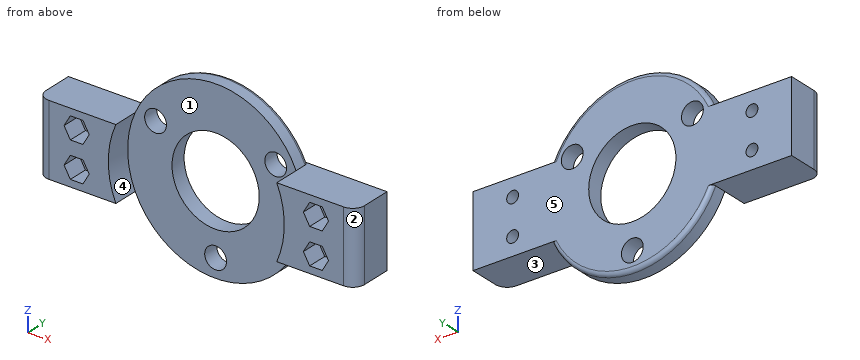
from build123d import *

# Parameters (mm, degrees)
SKETCH1_R                = 17.45
SKETCH1_R_2              = 12.45
BOSS_EXTRUDE1_DEPTH      = 8
SKETCH2_R                = 20
SKETCH2_R_2              = 12.45
BOSS_EXTRUDE2_DEPTH      = 2
SKETCH3_R                = 32.5
SKETCH3_R_2              = 12.45
BOSS_EXTRUDE3_DEPTH      = 4
FILLET1_R                = 1
BOSS_EXTRUDE6_START      = -4
SKETCH10_W               = 10
SKETCH10_H               = 18
BOSS_EXTRUDE6_DEPTH      = 4
SKETCH4_W                = 6
SKETCH4_H                = 18
BOSS_EXTRUDE4_DEPTH      = 75
BOSS_EXTRUDE4_DEPTH_BACK = 4
SKETCH5_R                = 5.05
CUT_EXTRUDE1_DEPTH       = 306
CUT_EXTRUDE1_DEPTH_BACK  = 113
SKETCH6_W                = 6
SKETCH6_H                = 10
BOSS_EXTRUDE5_DEPTH      = 15
BOSS_EXTRUDE5_DEPTH_BACK = 32.85
SKETCH7_R                = 1.629220746
SKETCH7_R_2              = 1.580258945
CUT_EXTRUDE2_DEPTH       = 10
SKETCH9_R                = 5.05
CUT_EXTRUDE3_DEPTH       = 10
CUT_EXTRUDE3_DEPTH_BACK  = 10
SKETCH11_W               = 9.782596874
SKETCH11_H               = 3.234517514
CUT_EXTRUDE4_DEPTH       = 123
CUT_EXTRUDE4_DEPTH_BACK  = 61
FILLET4_R                = 3
FILLET5_R                = 3
SKETCH12_W               = 108.791398151
SKETCH12_H               = 24.041848298
CUT_EXTRUDE5_DEPTH       = 110.678
SKETCH15_R               = 22
CUT_EXTRUDE7_DEPTH       = 4
SKETCH13_R               = 22
SKETCH13_R_2             = 11
SKETCH13_R_3             = 2.75
BOSS_EXTRUDE7_DEPTH      = 4
FILLET6_R                = 3
CUT_EXTRUDE8_DEPTH       = 5
FILLET7_R                = 1
BOSS_EXTRUDE8_START      = -3
BOSS_EXTRUDE8_DEPTH      = 9.4
FILLET8_R                = 3
FILLET8_OF_MIRROR2_R     = 3
CUT_EXTRUDE12_START      = -6
SKETCH21_R               = 6.05
CUT_EXTRUDE12_DEPTH      = 3.8
SKETCH18_W               = 88.746975794
SKETCH18_H               = 20.386854219
CUT_EXTRUDE9_DEPTH       = 10
SKETCH19_W               = 6
SKETCH19_H               = 10.45
BOSS_EXTRUDE9_DEPTH      = 5
FILLET9_R                = 2
CUT_EXTRUDE13_DEPTH      = 2
SKETCH23_R               = 1
CUT_EXTRUDE14_DEPTH      = 11
CUT_EXTRUDE16_DEPTH      = 1.7
SKETCH26_W               = 136.459260558
SKETCH26_H               = 86.542262852
CUT_EXTRUDE17_DEPTH      = 100
CUT_EXTRUDE17_DEPTH_BACK = 100
SKETCH27_R               = 1.5
CUT_EXTRUDE18_DEPTH      = 100
CUT_EXTRUDE19_DEPTH      = 5


with BuildPart() as part:
    # Sketch1 → Boss-Extrude1 (new body)
    with BuildSketch(Plane(origin=(0, 0, 0), x_dir=(1, 0, 0), z_dir=(0, 1, 0))):
        Circle(SKETCH1_R)
        Circle(SKETCH1_R_2, mode=Mode.SUBTRACT)
    extrude(amount=BOSS_EXTRUDE1_DEPTH)

    # Sketch2 → Boss-Extrude2 (add)
    with BuildSketch(Plane(origin=(0, 8, 0), x_dir=(1, 0, 0), z_dir=(0, 1, 0))):
        Circle(SKETCH2_R)
        Circle(SKETCH2_R_2, mode=Mode.SUBTRACT)
    extrude(amount=BOSS_EXTRUDE2_DEPTH)

    # Sketch3 → Boss-Extrude3 (add)
    with BuildSketch(Plane(origin=(0, 10, 0), x_dir=(1, 0, 0), z_dir=(0, 1, 0))):
        Circle(SKETCH3_R)
        Circle(SKETCH3_R_2, mode=Mode.SUBTRACT)
    extrude(amount=BOSS_EXTRUDE3_DEPTH)

    # Fillet1
    fillet1_edges = [part.edges().sort_by_distance(p)[0] for p in [
        (-32.5, 14, 0),
    ]]
    fillet(fillet1_edges, radius=FILLET1_R)

    # Sketch10 → Boss-Extrude6 (add)
    with BuildSketch(Plane(origin=(0, 14, 0), x_dir=(1, 0, 0), z_dir=(0, 1, 0)).offset(BOSS_EXTRUDE6_START)):
        with Locations((35.186917696, 0)):
            Rectangle(SKETCH10_W, SKETCH10_H)
        with Locations((-35.186917696, 0)):
            Rectangle(SKETCH10_W, SKETCH10_H)
    extrude(amount=BOSS_EXTRUDE6_DEPTH)

    # Sketch4 → Boss-Extrude4 (add, two sides)
    with BuildSketch(Plane(origin=(0, 14, 0), x_dir=(1, 0, 0), z_dir=(0, 1, 0))) as boss_extrude4_sk:
        with Locations((-37.186917696, 0)):
            Rectangle(SKETCH4_W, SKETCH4_H)
        with Locations((37.186917696, 0)):
            Rectangle(SKETCH4_W, SKETCH4_H)
    extrude(amount=BOSS_EXTRUDE4_DEPTH)
    extrude(boss_extrude4_sk.sketch, amount=-BOSS_EXTRUDE4_DEPTH_BACK)

    # Sketch5 → Cut-Extrude1 (cut, two sides)
    with BuildSketch(Plane.ZY.offset(-34.186917696)) as cut_extrude1_sk:
        with Locations((0, 79)):
            Circle(SKETCH5_R)
    extrude(amount=CUT_EXTRUDE1_DEPTH, mode=Mode.SUBTRACT)
    extrude(cut_extrude1_sk.sketch, amount=-CUT_EXTRUDE1_DEPTH_BACK, mode=Mode.SUBTRACT)

    # Sketch6 → Boss-Extrude5 (add, two sides)
    with BuildSketch(Plane(origin=(0, 0, -9), x_dir=(-1, 0, 0), z_dir=(0, 0, -1))) as boss_extrude5_sk:
        with Locations((37.186917696, 70.95)):
            Rectangle(SKETCH6_W, SKETCH6_H)
    extrude(amount=BOSS_EXTRUDE5_DEPTH)
    extrude(boss_extrude5_sk.sketch, amount=-BOSS_EXTRUDE5_DEPTH_BACK)

    # Sketch7 → Cut-Extrude2 (cut)
    with BuildSketch(Plane(origin=(-34.186917696, 0, 0), x_dir=(0, 0, -1), z_dir=(1, 0, 0))):
        with Locations((-17.5, 71)):
            Circle(SKETCH7_R)
        with Locations((17.5, 71)):
            Circle(SKETCH7_R_2)
    extrude(amount=-CUT_EXTRUDE2_DEPTH, mode=Mode.SUBTRACT)

    # Sketch9 → Cut-Extrude3 (cut, two sides)
    with BuildSketch(Plane(origin=(-34.186917696, 0, 0), x_dir=(0, 0, -1), z_dir=(1, 0, 0))) as cut_extrude3_sk:
        with Locations((0, 79)):
            Circle(SKETCH9_R)
    extrude(amount=CUT_EXTRUDE3_DEPTH, mode=Mode.SUBTRACT)
    extrude(cut_extrude3_sk.sketch, amount=-CUT_EXTRUDE3_DEPTH_BACK, mode=Mode.SUBTRACT)

    # Sketch11 → Cut-Extrude4 (cut, two sides)
    with BuildSketch(Plane.ZY.offset(-34.186917696)) as cut_extrude4_sk:
        with Locations((0, 15.617258757)):
            Rectangle(SKETCH11_W, SKETCH11_H)
    extrude(amount=CUT_EXTRUDE4_DEPTH, mode=Mode.SUBTRACT)
    extrude(cut_extrude4_sk.sketch, amount=-CUT_EXTRUDE4_DEPTH_BACK, mode=Mode.SUBTRACT)

    # Fillet4
    fillet4_edges = [part.edges().sort_by_distance(p)[0] for p in [
        (-37.186917696, 65.95, 23.85),
        (-37.186917696, 75.95, 23.85),
        (-37.186917696, 65.95, -24),
        (-37.186917696, 75.95, -24),
        (-37.186917696, 89, -9),
        (-37.186917696, 89, 9),
    ]]
    fillet(fillet4_edges, radius=FILLET4_R)

    # Fillet5
    fillet5_edges = [part.edges().sort_by_distance(p)[0] for p in [
        (40.186917696, 10, 0),
        (-40.186917696, 10, 0),
    ]]
    fillet(fillet5_edges, radius=FILLET5_R)

    # Sketch12 → Cut-Extrude5 (cut)
    with BuildSketch(Plane(origin=(40.186917696, 0, 0), x_dir=(0, 0, -1), z_dir=(1, 0, 0))):
        with Locations((-12.502918017, -2.020924149)):
            Rectangle(SKETCH12_W, SKETCH12_H)
    extrude(amount=-CUT_EXTRUDE5_DEPTH, mode=Mode.SUBTRACT)

    # Sketch15 → Cut-Extrude7 (cut)
    with BuildSketch(Plane(origin=(0, 14, 0), x_dir=(1, 0, 0), z_dir=(0, 1, 0))):
        Circle(SKETCH15_R)
    extrude(amount=-CUT_EXTRUDE7_DEPTH, mode=Mode.SUBTRACT)

    # Sketch13 → Boss-Extrude7 (add)
    with BuildSketch(Plane(origin=(0, 14, 0), x_dir=(1, 0, 0), z_dir=(0, 1, 0))):
        Circle(SKETCH13_R)
        Circle(SKETCH13_R_2, mode=Mode.SUBTRACT)
        with Locations((0, 17.5)):
            Circle(SKETCH13_R_3, mode=Mode.SUBTRACT)
        with Locations((-15.155444566, -8.75)):
            Circle(SKETCH13_R_3, mode=Mode.SUBTRACT)
        with Locations((15.155444566, -8.75)):
            Circle(SKETCH13_R_3, mode=Mode.SUBTRACT)
    extrude(amount=-BOSS_EXTRUDE7_DEPTH)

    # Fillet6
    fillet6_edges = [part.edges().sort_by_distance(p)[0] for p in [
        (37.186917696, 89, 9),
        (37.186917696, 89, -9),
    ]]
    fillet(fillet6_edges, radius=FILLET6_R)

    # Sketch16 → Cut-Extrude8 (cut)
    with BuildSketch(Plane.XZ.offset(-10)):
        with BuildLine():
            Line((-31.228992939, 9), (-20.29384143, 9))
            ThreePointArc((-20.29384143, 9), (0, 22.2), (20.29384143, 9))
            Line((20.29384143, 9), (31.228992939, 9))
            ThreePointArc((31.228992939, 9), (0, 32.5), (-31.228992939, 9))
        make_face()
    cut_extrude8 = extrude(amount=-CUT_EXTRUDE8_DEPTH, mode=Mode.SUBTRACT)

    # Mirror1: Cut-Extrude8 across plane
    add(cut_extrude8.mirror(Plane.XY), mode=Mode.SUBTRACT)

    # Fillet7
    fillet7_edges = [part.edges().sort_by_distance(p)[0] for p in [
        (0, 14, 22.2),
        (0, 14, -22.2),
    ]]
    fillet(fillet7_edges, radius=FILLET7_R)

    # Sketch17 → Boss-Extrude8 (add)
    with BuildSketch(Plane.XZ.offset(-10).offset(BOSS_EXTRUDE8_START)):
        with BuildLine():
            Line((20.29384143, -9), (40.186917696, -9))
            Line((40.186917696, -9), (40.186917696, 9))
            Line((40.186917696, 9), (20.29384143, 9))
            ThreePointArc((20.29384143, 9), (22.2, 0), (20.29384143, -9))
        make_face()
    boss_extrude8 = extrude(amount=BOSS_EXTRUDE8_DEPTH)

    # Fillet8
    fillet8_edges = [part.edges().sort_by_distance(p)[0] for p in [
        (40.186917696, 3.6, 0),
    ]]
    fillet(fillet8_edges, radius=FILLET8_R)

    # Mirror2: Boss-Extrude8 across plane
    add(boss_extrude8.mirror(Plane(origin=(0, 0, 0), x_dir=(0, 0, 1), z_dir=(1, 0, 0))))

    # Fillet8 of Mirror2
    fillet8_of_mirror2_edges = [part.edges().sort_by_distance(p)[0] for p in [
        (-40.186917696, 3.6, 0),
    ]]
    fillet(fillet8_of_mirror2_edges, radius=FILLET8_OF_MIRROR2_R)

    # Sketch21 → Cut-Extrude12 (cut)
    with BuildSketch(Plane(origin=(40.186917696, 0, 0), x_dir=(0, 0, -1), z_dir=(1, 0, 0)).offset(CUT_EXTRUDE12_START)):
        with Locations((0, 79)):
            Circle(SKETCH21_R)
    extrude(amount=CUT_EXTRUDE12_DEPTH, mode=Mode.SUBTRACT)

    # Sketch18 → Cut-Extrude9 (cut)
    with BuildSketch(Plane(origin=(40.186917696, 0, 0), x_dir=(0, 0, -1), z_dir=(1, 0, 0))):
        with Locations((0, 89.193427109)):
            Rectangle(SKETCH18_W, SKETCH18_H)
    extrude(amount=-CUT_EXTRUDE9_DEPTH, mode=Mode.SUBTRACT)

    # Sketch19 → Boss-Extrude9 (add)
    with BuildSketch(Plane(origin=(0, 79, 0), x_dir=(1, 0, 0), z_dir=(0, 1, 0))):
        with Locations((37.186917696, -11.275)):
            Rectangle(SKETCH19_W, SKETCH19_H)
        with Locations((37.186917696, 11.275)):
            Rectangle(SKETCH19_W, SKETCH19_H)
    extrude(amount=-BOSS_EXTRUDE9_DEPTH)

    # Fillet9
    fillet9_edges = [part.edges().sort_by_distance(p)[0] for p in [
        (37.186917696, 74, 16.5),
        (37.186917696, 74, -16.5),
    ]]
    fillet(fillet9_edges, radius=FILLET9_R)

    # Sketch22 → Cut-Extrude13 (cut)
    with BuildSketch(Plane(origin=(-34.186917696, 0, 0), x_dir=(0, 0, -1), z_dir=(1, 0, 0))):
        Polygon((-15.9988893, 68.4), (-14.4977786, 71), (-15.9988893, 73.6), (-19.0011107, 73.6), (-20.5022214, 71), (-19.0011107, 68.4), align=None)
        Polygon((20.5022214, 71), (19.0011107, 73.6), (15.9988893, 73.6), (14.4977786, 71), (15.9988893, 68.4), (19.0011107, 68.4), align=None)
    extrude(amount=-CUT_EXTRUDE13_DEPTH, mode=Mode.SUBTRACT)

    # Sketch23 → Cut-Extrude14 (cut)
    with BuildSketch(Plane(origin=(0, 79, 0), x_dir=(1, 0, 0), z_dir=(0, 1, 0))):
        with Locations((37.186917696, -12.3)):
            Circle(SKETCH23_R)
        with Locations((37.186917696, 12.3)):
            Circle(SKETCH23_R)
    extrude(amount=-CUT_EXTRUDE14_DEPTH, mode=Mode.SUBTRACT)

    # Sketch24 → Cut-Extrude16 (cut)
    with BuildSketch(Plane.XZ.offset(-74)):
        Polygon((37.186917696, 9.990598923), (39.186917696, 11.145299462), (39.186917696, 13.454700538), (37.186917696, 14.609401077), (35.186917696, 13.454700538), (35.186917696, 11.145299462), align=None)
        Polygon((37.186917696, -14.609401077), (39.186917696, -13.454700538), (39.186917696, -11.145299462), (37.186917696, -9.990598923), (35.186917696, -11.145299462), (35.186917696, -13.454700538), align=None)
    extrude(amount=-CUT_EXTRUDE16_DEPTH, mode=Mode.SUBTRACT)

    # Sketch26 → Cut-Extrude17 (cut, two sides)
    with BuildSketch(Plane(origin=(0, 0, -9), x_dir=(-1, 0, 0), z_dir=(0, 0, -1))) as cut_extrude17_sk:
        with Locations((-1.263679096, 57.271131426)):
            Rectangle(SKETCH26_W, SKETCH26_H)
    extrude(amount=CUT_EXTRUDE17_DEPTH, mode=Mode.SUBTRACT)
    extrude(cut_extrude17_sk.sketch, amount=-CUT_EXTRUDE17_DEPTH_BACK, mode=Mode.SUBTRACT)

    # Sketch27 → Cut-Extrude18 (cut)
    with BuildSketch(Plane(origin=(0, 14, 0), x_dir=(1, 0, 0), z_dir=(0, 1, 0))):
        with Locations((30.186917696, -4.5)):
            Circle(SKETCH27_R)
        with Locations((30.186917696, 4.5)):
            Circle(SKETCH27_R)
        with Locations((-30.186917696, -4.5)):
            Circle(SKETCH27_R)
        with Locations((-30.186917696, 4.5)):
            Circle(SKETCH27_R)
    extrude(amount=-CUT_EXTRUDE18_DEPTH, mode=Mode.SUBTRACT)

    # Sketch28 → Cut-Extrude19 (cut)
    with BuildSketch(Plane.XZ.offset(-3.6)):
        Polygon((27.011491216, -4.5), (28.599204456, -7.25), (31.774630937, -7.25), (33.362344177, -4.5), (31.774630937, -1.75), (28.599204456, -1.75), align=None)
        Polygon((27.011491216, 4.5), (28.599204456, 1.75), (31.774630937, 1.75), (33.362344177, 4.5), (31.774630937, 7.25), (28.599204456, 7.25), align=None)
        Polygon((-33.362344177, 4.5), (-31.774630937, 1.75), (-28.599204456, 1.75), (-27.011491216, 4.5), (-28.599204456, 7.25), (-31.774630937, 7.25), align=None)
        Polygon((-33.362344177, -4.5), (-31.774630937, -7.25), (-28.599204456, -7.25), (-27.011491216, -4.5), (-28.599204456, -1.75), (-31.774630937, -1.75), align=None)
    extrude(amount=-CUT_EXTRUDE19_DEPTH, mode=Mode.SUBTRACT)


solid = part.part
Geometry check sheet. Reference: the model listing, model coordinates, mm. Face numbers are marked on the shaded views. A direction names the side the tool comes from. Coordinates: 2 decimals unless noted, no trailing zeros. Order: outer loops, then holes, each group sorted by start corner. A loop starts at its lowest first (then second) coordinate and runs counter-clockwise, first axis right, second up. Notation, with made-up numbers: (7.5, 30.25) -> (61.5, 30.25) arc R15 cw to (61.5, 47.25) -> close; hole circle Ø4 at (31, -15.5). An arc over 180 degrees is marked (long way). Use a Markdown table: item, result. Add a question column.
1. Cross-section at B-B (x = 0). Enter the section's corners in (y, z), and give its area (3 significant figures).
2. Cross-section at C-C (z = 0). Enter the section's corners in (x, y), and give its area (3 significant figures).
3. Go/stop test with flat-tipped pins: pin 1 Ø4 at (x, z) = (30.19, -4.5) entering from +Y; pin 2 Ø3.5 at (x, y) = (30.5, 6.5) entering from +Z; pin 3 Ø3.5 at (x, y) = (29.5, 5.5) entering from -Z; pin 4 Ø1 at (x, y) = (0, 10.5) entering from -Z. Record where each tip stops, or that it passes through.
4. Mould release check, pull along X, two halves, no side actions. Record for the marked faces 1, 2 and 3: pulls with the +X half, pulls with the -X half, needs draft (parallel to the pull), parting line crosses it, or undercut.
5. Set-up check for the marked faces 4 and 5: record each of +Z, -Z, +X, -X, +Y, -Y from which the full face is reachable in a straight line by a thin tool's end or side.
6. Material ranges on L1, parallel to X at y = 4, z = 2.5; L2, parallel to X at y = 11.65, z = -4.5; L3, parallel to X at y = 12.55, z = 0, recorded low to high.
7. Cross-section at A-A (y = 7.5). Give the number of separate pieces and of enclosed holes in the cut face, and give its area (3 significant figures).
Filled sheet:
| question | item | result |
|---|---|---|
| 1 | outline | (10, -22.2) -> (13, -22.2) arc R1 ccw to (14, -21.2) -> (14, -20.25) -> (10, -20.25) -> close; (10, -14.75) -> (14, -14.75) -> (14, -11) -> (10, -11) -> close; (10, 11) -> (14, 11) -> (14, 21.2) arc R1 ccw to (13, 22.2) -> (10, 22.2) -> close |
| 1 | area | 67.2 mm2 |
| 2 | outline | (-40.19, 6.6) arc R3 ccw to (-37.19, 3.6) -> (-22.2, 3.6) -> (-22.2, 10) -> (-11, 10) -> (-11, 14) -> (-40.19, 14) -> close; (11, 10) -> (22.2, 10) -> (22.2, 3.6) -> (37.19, 3.6) arc R3 ccw to (40.19, 6.6) -> (40.19, 14) -> (11, 14) -> close |
| 2 | area | 460 mm2 |
| 3 | pin 1 | y = 14 |
| 3 | pin 2 | z = 9 |
| 3 | pin 3 | z = -9 |
| 3 | pin 4 | z = -22.2 |
| 4 | face 1 | undercut |
| 4 | face 2 | pulls with the +X half |
| 4 | face 3 | needs draft |
| 5 | face 4 | -Y |
| 5 | face 5 | +Z, -Z, +X, -X, +Y |
| 6 | L1 | -38.68 to -32.21, -28.17 to -22.06, 22.06 to 28.17, 32.21 to 38.68 |
| 6 | L2 | -40.19 to -31.69, -28.69 to -10.04, 10.04 to 28.69, 31.69 to 40.19 |
| 6 | L3 | -40.19 to -11, 11 to 40.19 |
| 7 | separate pieces | 2 |
| 7 | enclosed holes | 4 |
| 7 | area | 565 mm2 |
